from build123d import *

# Parameters (mm, degrees)
SALIENTE_EXTRUIR1_DEPTH = 3
CROQUIS2_R              = 38.5
CROQUIS2_R_2            = 2.25
CROQUIS2_R_3            = 1.6
CORTAR_EXTRUIR1_DEPTH   = 3


with BuildPart() as part:
    # Croquis1 → Saliente-Extruir1 (new body)
    with BuildSketch(Plane.XY):
        Polygon((-261.838674033, 298.703267526), (-260.838674033, 298.703267526), (-260.838674033, 323.703267526), (187.161325967, 323.703267526), (187.161325967, 298.703267526), (188.161325967, 298.703267526), (188.161325967, -197.096732474), (-261.838674033, -197.096732474), align=None)
    extrude(amount=SALIENTE_EXTRUIR1_DEPTH)

    # Croquis2 → Cortar-Extruir1 (cut)
    with BuildSketch(Plane.XY.offset(3)):
        with Locations((-143.338674033, -58.596732474)):
            Circle(CROQUIS2_R)
        with Locations((-107.488674033, -22.746732474)):
            Circle(CROQUIS2_R_2)
        with Locations((-107.488674033, -94.446732474)):
            Circle(CROQUIS2_R_2)
        with Locations((-179.188674033, -94.446732474)):
            Circle(CROQUIS2_R_2)
        with Locations((-179.188674033, -22.746732474)):
            Circle(CROQUIS2_R_2)
        with Locations((-93.338674033, -8.596732474)):
            Circle(CROQUIS2_R_3)
        with Locations((-93.338674033, -108.596732474)):
            Circle(CROQUIS2_R_3)
        with Locations((-193.338674033, -108.596732474)):
            Circle(CROQUIS2_R_3)
        with Locations((-193.338674033, -8.596732474)):
            Circle(CROQUIS2_R_3)
    extrude(amount=-CORTAR_EXTRUIR1_DEPTH, mode=Mode.SUBTRACT)


solid = part.part
Geometry check sheet. Reference: the model listing, model coordinates, mm. Coordinates: 2 decimals unless noted, no trailing zeros. Order: outer loops, then holes, each group sorted by start corner. A loop starts at its lowest first (then second) coordinate and runs counter-clockwise, first axis right, second up. Notation, with made-up numbers: M 89.5,53 L 116.5,53 A17 ccw 116.5,79 Z; hole C -18.75,9 d10. An arc over 180 degrees is marked long. Use CSV: the item, a comma, the result in double quotes.
Item 1: Cross-section at A-A on x = -153.5. Record the cut outline in (y, z), then the cut area to 3 significant figures.
Returned:
outline,"M -197.1,0 L -95.73,0 L -95.73,3 L -197.1,3 Z; M -21.46,0 L 323.7,0 L 323.7,3 L -21.46,3 Z"
area,"1,340 mm2"
Item 2: Mould release check, pull along X, two halves, no side actions. Record for faces 1 (the flat face through (-34, 67, 0)), 2 (the cylindrical face through (-106.617, -47.032, 1.521)): pulls with the +X half, pulls with the -X half, needs draft (parallel to the pull), parting line crosses it, or undercut.
Returned:
face 1,"needs draft"
face 2,"undercut"
Item 3: Cross-section at B-B on z = 0.6. Give the number of separate pieces and of enclosed holes in the cut face, then the cut area to 3 significant figures.
Returned:
separate pieces,"1"
enclosed holes,"9"
area,"230,000 mm2"
Item 4: Gauge pin test, flat ends, axial feed: pin 1 Ø5 at (x, y) = (-193.34, -108.6) entering from -Z; pin 2 Ø1.1 at (x, z) = (188, 2) entering from +Y; pin 3 Ø0.9 at (y, z) = (315, 1.5) entering from +X. Record the tip position at first contact, or that the pin passes through.
Returned:
pin 1,"stops at z = 0"
pin 2,"stops at y = 298.7"
pin 3,"stops at x = 187.16"
Item 5: Thickness scan on line 1 along X through (y, z) = (-43.5, 2.1); line 2 along Y through (x, z) = (-111.5, 0.5); line 3 along Y through (x, z) = (-174.5, 1.35). Record the ranges inside material, lowest first.
Returned:
line 1,"x = -261.84 to -178.76, -107.92 to 188.16"
line 2,"y = -197.1 to -80.24, -36.95 to 323.7"
line 3,"y = -197.1 to -81.21, -35.99 to 323.7"
